```python
from build123d import *

# Parameters (mm, degrees)
FILLET1_R          = 5
CUT_EXTRUDE1_START = -10
CUT_EXTRUDE1_DEPTH = 10


with BuildPart() as part:
    # Sketch1 → Revolve1 (revolve)
    with BuildSketch(Plane(origin=(0, 0, 0), x_dir=(1, 0, 0), z_dir=(0, 1, 0))):
        Polygon((5.5, 14.5), (0, 14.5), (0, -369.5), (5.5, -369.5), (6, -369), (6, -357.5), (12.5, -357.5), (12.5, -355), (25, -355), (25, 0), (12.5, 0), (12.5, 2.5), (6, 2.5), (6, 14), align=None)
    revolve(axis=Axis((0, 0, -14.5), (0, 0, 1)))

    # Fillet1
    fillet1_edges = [part.edges().sort_by_distance(p)[0] for p in [
        (-25, 0, 355),
        (-25, 0, 0),
    ]]
    fillet(fillet1_edges, radius=FILLET1_R)

    # Sketch2 → Cut-Extrude1 (cut)
    with BuildSketch(Plane.XY.offset(369.5).offset(CUT_EXTRUDE1_START)):
        with BuildLine():
            ThreePointArc((4.472135955, 4), (0, 6), (-4.472135955, 4))
            Line((-4.472135955, 4), (4.472135955, 4))
        make_face()
        with BuildLine():
            Line((4.472135955, -4), (-4.472135955, -4))
            ThreePointArc((-4.472135955, -4), (0, -6), (4.472135955, -4))
        make_face()
    extrude(amount=CUT_EXTRUDE1_DEPTH, mode=Mode.SUBTRACT)


solid = part.part
```
For this review, take the finished solid that the model builds, in its own axes (mm). A direction names the side the tool comes from. Round coordinates to 2 decimals unless told otherwise and drop trailing zeros. Loops run counter-clockwise (first coordinate to the right, second up) from the corner with the lowest first, then second, coordinate; pieces in that order, holes last.
Q1. Insertion check: pin 1 Ø4 at (y, z) = (7, 230) entering from +X; pin 2 Ø8 at (y, z) = (14.5, 129) entering from +X; pin 3 Ø4.5 at (x, z) = (-2, 363) entering from +Y. Each pin has a flat end and moves straight along its axis. Give the tip position at first contact, or say it passes through.
Result sheet:
pin 1: stops at x = 24.49
pin 2: stops at x = 22.69
pin 3: stops at y = 4
Q2. Machinability: for faces 1 (the face through (0, 4, 364)), 2 (the face through (11.923, 3.755, -1.268)), 3 (the face through (23.846, 7.509, 175.085)), 4 (the face through (0, -4, 364)), 5 (the face through (-9, 9, 355)), which of the approach directions +Z, -Z, +X, -X, +Y, -Y give a long, thin tool a straight path to every point of the face, cutting with its end or side? Answer none if there is none.
Result sheet:
face 1: +Z, +X, -X, +Y
face 2: -Z
face 3: +Z, -Z
face 4: +Z, +X, -X, -Y
face 5: +Z
Q3. Add section B-B on z = 200. Write out the cut boundary in (x, y), plus the area to 3 significant figures.
Result sheet:
outline: circle Ø50 at (0, 0)
area: 1,960 mm2
Q4. To check wall thickness, follow line 1 along Z through (x, y) = (-3, 17.5); line 2 along X through (y, z) = (-15, 86); line 3 along Y through (x, z) = (0.5, 155) (3 decimals). State the ranges of each line that lie inside material, in increasing order.
Result sheet:
line 1: z = 0 to 355
line 2: x = -20 to 20
line 3: y = -24.995 to 24.995
